Can you work these out from the model? Positions are in its coordinate system, mm. A direction names the side the tool comes from. Round coordinates to 2 decimals unless told otherwise and drop trailing zeros. Order: outer loops, then holes, each group sorted by start corner. A loop starts at its lowest first (then second) coordinate and runs counter-clockwise, first axis right, second up. Notation, with made-up numbers: (-30.75, 14) - (-24.75, 14) arc R25 cw to (-24.75, 38) - close; hole circle Ø5 at (39.25, 55.5). An arc over 180 degrees is marked (long way). Write item = value, one per line.
from build123d import *

# Parameters (mm, degrees)
SKETCH1_R           = 5
BOSS_EXTRUDE1_DEPTH = 5
FILLET1_R           = 5


with BuildPart() as part:
    # Sketch1 → Boss-Extrude1 (new body)
    with BuildSketch(Plane.XY):
        with BuildLine():
            Line((0, 0), (30, 0))
            Line((30, 0), (50, 20))
            Line((50, 20), (50, 40))
            Line((50, 40), (30, 40))
            Line((30, 40), (30, 35))
            ThreePointArc((30, 35), (27.071067812, 27.928932188), (20, 25))
            Line((20, 25), (10, 25))
            ThreePointArc((10, 25), (2.928932188, 27.928932188), (0, 35))
            Line((0, 35), (0, 40))
            Line((0, 40), (-20, 40))
            Line((-20, 40), (-20, 20))
            Line((-20, 20), (0, 0))
        make_face()
        with Locations((-10, 30)):
            Circle(SKETCH1_R, mode=Mode.SUBTRACT)
        with Locations(Location((40, 30, 0), (0, 0, 180))):
            Circle(SKETCH1_R, mode=Mode.SUBTRACT)
    extrude(amount=BOSS_EXTRUDE1_DEPTH)

    # Fillet1
    fillet1_edges = [part.edges().sort_by_distance(p)[0] for p in [
        (50, 40, 2.5),
        (-20, 40, 2.5),
    ]]
    fillet(fillet1_edges, radius=FILLET1_R)


solid = part.part
(1) On a 3-axis mill with a long thin cutter (end or side, diameter ignored), from which of +Z, -Z, +X, -X, +Y, -Y can I reach the whole of each face in a straight line? I mean faces 1 (the face through (0, 37, 2)), 2 (the face through (45, 30, 2)). Say none if no direction works.
Computed:
face_1 = +Z, -Z, +Y
face_2 = +Z, -Z
(2) If we section it at D-D (y = 14): Write out the boundary of the cut face in (x, z), plus the area to 3 significant figures.
Computed:
outline = (-14, 0) - (44, 0) - (44, 5) - (-14, 5) - close
area = 290 mm^2
(3) If we section it at C-C (y = 30): Write out the boundary of the cut face in (x, z), plus the area to 3 significant figures.
Computed:
outline = (-20, 0) - (-15, 0) - (-15, 5) - (-20, 5) - close; (-5, 0) - (1.34, 0) - (1.34, 5) - (-5, 5) - close; (28.66, 0) - (35, 0) - (35, 5) - (28.66, 5) - close; (45, 0) - (50, 0) - (50, 5) - (45, 5) - close
area = 113 mm^2
(4) Will these pins go through, and if not, where does the flat tip stop? P1, Ø6, axis at x = 40, y = 30, coming from the -Z side; P2, Ø1.5, axis at x = 17, z = 3.5, coming from the +Y side.
Computed:
P1 = through
P2 = 25
(5) Thinking about a two-plate mould opening in X: for faces 3 (the face through (40, 10, 2)), 4 (the face through (-5.381, 28.085, 2.465)), 5 (the face through (15, 20, 0)), which applies, +X half, -X half, draft (parallel to the pull), parting line (faces both ways), or undercut?
Computed:
face_3 = +X half
face_4 = undercut
face_5 = draft
(6) If we section it at B-B (z = 1.3): Write out the boundary of the cut face in (x, y), plus the area to 3 significant figures.
Computed:
outline = (-20, 20) - (0, 0) - (30, 0) - (50, 20) - (50, 35) arc R5 ccw to (45, 40) - (30, 40) - (30, 35) arc R10 cw to (20, 25) - (10, 25) arc R10 cw to (0, 35) - (0, 40) - (-15, 40) arc R5 ccw to (-20, 35) - close; hole circle Ø10 at (-10, 30); hole circle Ø10 at (40, 30)
area = 1,830 mm^2
(7) If I drill on line 1 (Y direction, x = -10, z = 1.7); line 2 (X direction, y = 29, z = 1.3); line 3 (X direction, y = 32.5, z = 2.25), over which ranges is the centre line in solid material (lowest first)? Write a range as from..to.
Computed:
line_1 = 10..25, 35..40
line_2 = -20..-14.9, -5.1..2, 28..35.1, 44.9..50
line_3 = -20..-14.33, -5.67..0.32, 29.68..35.67, 44.33..50
(8) If we section it at A-A (x = -10): Write out the boundary of the cut face in (y, z).
Computed:
outline = (10, 0) - (25, 0) - (25, 5) - (10, 5) - close; (35, 0) - (40, 0) - (40, 5) - (35, 5) - close
